```python
from build123d import *

# Parameters (mm, degrees)
F0_R     = 19.05
F1_DEPTH = 101.6
F3_D     = 6.35
F4_R     = 25.402508
F5_DEPTH = 25.4
F6_R     = 6.35
F7_DEPTH = 25.4
F8_R     = 6.35
F9_DEPTH = 127
F10_R    = 5.08


with BuildPart() as f1:
    # F0 (on Top) → F1 (new body)
    with BuildSketch(Plane.XY):
        Circle(F0_R)
    extrude(amount=F1_DEPTH)

    # F3 (through all)
    with Locations(Plane(origin=(0, 0, 0), x_dir=(1, 0, 0), z_dir=(0, 0, -1))):
        with Locations((0, 0)):
            Hole(F3_D / 2)

    # F4 (on face) → F5 (join)
    with BuildSketch(Plane.XY.offset(101.6)):
        Circle(F4_R)
    extrude(amount=F5_DEPTH)

    # F6 (on Front) → F7 (cut)
    with BuildSketch(Plane.XZ):
        with Locations((0, 114.860535)):
            Circle(F6_R)
    extrude(amount=F7_DEPTH, mode=Mode.SUBTRACT)

    # F8 (on face) → F9 (cut)
    with BuildSketch(Plane.XZ):
        with Locations((0, 114.860535)):
            Circle(F8_R)
    extrude(amount=F9_DEPTH, mode=Mode.SUBTRACT)

    # F10
    f10_edges = [f1.edges().sort_by_distance(p)[0] for p in [
        (-25.402508, 0, 101.6),
        (-25.402508, 0, 127),
    ]]
    fillet(f10_edges, radius=F10_R)


solid = f1.part
```
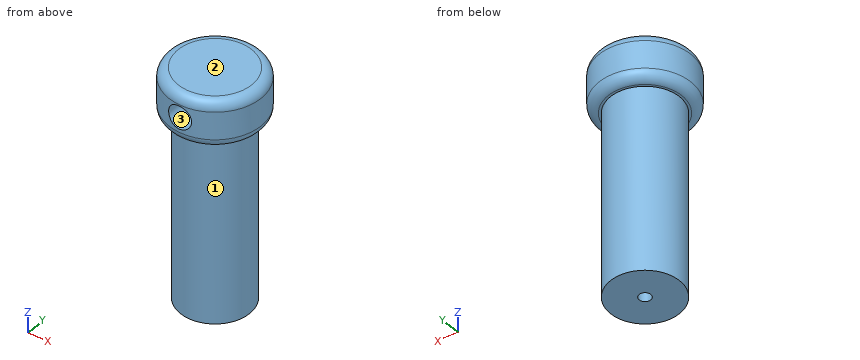
CAD build for the part. Positions are in the model's coordinates, mm. Face numbers are marked on the shaded views. Round coordinates to 2 decimals unless told otherwise and drop trailing zeros. Order: outer loops, then holes, each group sorted by start corner. A loop starts at its lowest first (then second) coordinate and runs counter-clockwise, first axis right, second up.
Q1. Wall check: L1, parallel to Z at x = 0, y = -12; L2, parallel to Y at x = 0, z = 26 (3 decimals); L3, parallel to Z at x = -19, y = -8. Give the ranges that are in metal, low to high.
Q2. Slice it at A-A (z = 33). Write the cut outline in (x, y) (3 decimals).
Q3. Two-plate mould, pull along X, no slides. Class the marked faces 1, 2 and 3: pulls with the +X half, pulls with the -X half, needs draft (parallel to the pull), parting line crosses it, or undercut.
Q4. Drop flat-ended pins along their axis: pin 1 (12 mm diameter, centred on y = 12, z = 19, fed in from +X); pin 2 (1.9 mm diameter, centred on x = -1, y = 0.5, fed in from -Z); pin 3 (6 mm diameter, centred on x = -8, z = 83.5, fed in from -Y); pin 4 (10 mm diameter, centred on x = -2, z = 118, fed in from -Y). Give the stop position or say it passes through.
Results below:
1. L1: z = 0 to 108.51, 121.21 to 127
1. L2: y = -19.05 to -3.175, 3.175 to 19.05
1. L3: z = 101.61 to 126.99
2. outline: circle Ø38.1 at (0, 0); hole circle Ø6.35 at (0, 0)
3. face 1: parting line crosses it
3. face 2: needs draft
3. face 3: undercut
4. pin 1: stops at x = 18.08
4. pin 2: stops at z = 101.6
4. pin 3: stops at y = -18.38
4. pin 4: stops at y = -25.4
